Geometry: final body of the model. Coordinates: model frame, mm. A direction names the side the tool comes from. Give positions to 0.01 mm unless a question says otherwise; leave off trailing zeros. Loops run counter-clockwise (first coordinate to the right, second up) from the corner with the lowest first, then second, coordinate; pieces in that order, holes last. Notation, with made-up numbers: (68, 88.5) - (127, 88.5) arc R27 ccw to (127, 112.5) - close; hole circle Ø6 at (-32, 21.5). An arc over 180 degrees is marked (long way). Use one line per item in the form item = value.
Autodesk Inventor part; units mm, degrees
ref_plane "YZ Plane" through (0, 0, 0) normal (1, 0, 0) x (0, 1, 0)
ref_plane "XZ Plane" through (0, 0, 0) normal (0, 1, 0) x (-1, 0, 0)
ref_plane "XY Plane" through (0, 0, 0) normal (0, 0, 1) x (1, 0, 0)
sketch "Sketch1" plane through (0, 0, 0) normal (0, 0, 1) x (1, 0, 0)
  line L0 (0, 0) -> (0, 87.5)
  line L1 (0, 87.5) -> (43.6046, 111.967)
  line L2 (0, 0) -> (50, 0)
  line L3 (50, 0) -> (93.217, 25.1454)
  circle A0 centre (68.0717, 68.3624) radius 50 construction
  arc A1 (93.217, 25.1454) -> (43.6046, 111.967) centre (68.0717, 68.3624) ccw
  dimension "d0" = 87.5
  dimension "d1" = 50
  dimension "d2" = 50
  dimension "d3" = 50
  dimension "d4" = 100
extrude "Extrusion1" add sketch "Sketch1" along normal blind 50
sketch "Sketch2" plane through (0, 0, 50) normal (0, 0, 1) x (1, 0, 0)
  line L0 (0, 0) -> (50, 0)
  line L1 (50, 0) -> (93.217, 25.1454)
  arc A0 (93.217, 25.1454) -> (43.6046, 111.967) centre (68.0717, 68.3624) ccw
  line L2 (43.6046, 111.967) -> (0, 87.5)
  line L3 (0, 81.7667) -> (46.0513, 107.6066)
  arc A1 (90.7025, 29.4671) -> (46.0513, 107.6066) centre (68.0717, 68.3624) ccw
  line L4 (90.7025, 29.4671) -> (48.6512, 5)
  line L5 (48.6512, 5) -> (0, 5)
  line L6 (0, 87.5) -> (0, 0)
  line L7 (0, 5) -> (0, 81.7667)
  dimension "d7" = 5
extrude "Extrusion2" cut sketch "Sketch2" against normal blind 45 contours L6 L3 A1 L4 L5
sketch "Sketch3" plane through (0, 0, 0) normal (-1, 0, 0) x (0, 0, 1)
  line L0 (0, 87.5) -> (50, 87.5)
  line L1 (50, 113.3624) -> (50, 29.4671)
  line L2 (0, 87.5) -> (50, 87.5)
  line L3 (50, 87.5) -> (50, 72.5)
  line L4 (50, 72.5) -> (0, 72.5)
  line L5 (0, 72.5) -> (0, 87.5)
  point P0 (0, 0)
  point P1 (50, 107.6066)
  dimension "d10" = 15
extrude "Extrusion3" add sketch "Sketch3" against normal blind 5
sketch "Sketch4" plane through (0, 0, 0) normal (-1, 0, 0) x (0, 0, 1)
  line L0 (0, 87.5) -> (0, 111.967)
  line L1 (0, 87.5) -> (15, 87.5)
  line L2 (15, 87.5) -> (15, 32.5)
  line L3 (15, 32.5) -> (0, 32.5)
  line L4 (0, 32.5) -> (0, 87.5)
  line L5 (0, 0) -> (50, 0)
  dimension "d13" = 15
  dimension "d14" = 32.5
extrude "Extrusion4" add sketch "Sketch4" against normal blind 5
sketch "Sketch5" plane through (0, 0, 5) normal (0, 0, 1) x (1, 0, 0)
  circle A0 centre (25, 27.5) radius 5
  line L0 (0, 0) -> (50, 0)
  dimension "d17" = 10
  dimension "d18" = 27.5
  dimension "d19" = 25
extrude "Extrusion5" add sketch "Sketch5" along normal blind 90
sketch "Sketch6" plane through (0, 0, 5) normal (0, 0, 1) x (1, 0, 0)
  circle A0 centre (25, 27.5) radius 5
  circle A1 centre (25, 27.5) radius 20
  point P0 (0, 0)
  dimension "d22" = 40
extrude "Extrusion6" add sketch "Sketch6" along normal blind 10
sketch "Sketch7" plane through (0, 0, 5) normal (0, 0, 1) x (1, 0, 0)
  arc A0 (93.217, 25.1454) -> (43.6046, 111.967) centre (68.0717, 68.3624) ccw
  circle A1 centre (68.0717, 68.3624) radius 6.25
  circle A2 centre (68.0717, 68.3624) radius 21.25
  point P0 (0, 0)
  dimension "d25" = 12.5
  dimension "d28" = 15
extrude "Extrusion8" add sketch "Sketch7" along normal blind 10
sketch "Sketch8" plane through (68.0717, 68.3624, 5) normal (0, 0, 1) x (1, 0, 0)
  circle A0 centre (0, 0) radius 6.25
  circle A1 centre (0, 0) radius 6.25
  point P0 (-68.0717, -68.3624)
extrude "Extrusion9" cut sketch "Sketch8" against normal through all
sketch "Sketch9" plane through (0, 0, 0) normal (0, 0, -1) x (-1, 0, 0)
  circle A0 centre (-68.0717, 68.3624) radius 21.25
  circle A1 centre (-68.0717, 68.3624) radius 21.25
  point P0 (0, 0)
extrude "Extrusion10" add sketch "Sketch9" along normal blind 5
sketch "Sketch10" plane through (0, 0, 50) normal (0, 0, 1) x (1, 0, 0)
  arc A0 (93.217, 25.1454) -> (43.6046, 111.967) centre (68.0717, 68.3624) ccw
  circle A1 centre (68.0717, 68.3624) radius 50
  line L0 (18.0717, 68.3624) -> (18.0717, 97.6402)
  line L1 (0, 87.5) -> (43.6046, 111.967)
  line L2 (43.6046, 111.967) -> (18.0717, 97.6402)
  line L3 (68.0717, 18.3624) -> (81.5592, 18.3624)
  line L4 (50, 0) -> (93.217, 25.1454)
  line L5 (81.5592, 18.3624) -> (93.217, 25.1454)
  point P0 (0, 0)
extrude "Extrusion11" cut sketch "Sketch10" against normal blind 10
properties part number "BA005" material "ABS Plastic"
(1) Pin query (flat end, axial travel): P1, Ø1.5, axis at x = 88.5, y = 98, coming from the -Z side; P2, Ø8, axis at x = 57, z = 41, coming from the +Y side; P3, Ø3, axis at x = 74.5, z = 45, coming from the +Y side. Return the tip coordinate at first contact, or that it passes through.
Solution:
P1 = 0
P2 = 117.84
P3 = 18.36
(2) Pull-direction query (X, two-part tool) for faces 1 (the face through (111, 94, 20)), 2 (the face through (25.24, 95.93, 22.82)), 3 (the face through (0, 43, 14)); classes: released by +X, released by -X, zero draft, split by the parting line, or undercut.
Solution:
face_1 = split by the parting line
face_2 = undercut
face_3 = released by -X
(3) Cut plane C-C (y = 27.5). Return the cut outline in (x, z), plus the area to 3 significant figures.
Solution:
outline = (0, 0) - (96.89, 0) - (96.89, 40) - (87.32, 40) - (87.32, 5) - (45, 5) - (45, 15) - (30, 15) - (30, 95) - (20, 95) - (20, 15) - (5, 15) - (5, 5) - (0, 5) - close
area = 2,020 mm2
(4) Cut plane B-B (x = 55). Return the cut outline in (y, z), plus the area to 3 significant figures.
Solution:
outline = (2.91, 0) - (51.61, 0) - (51.61, -5) - (85.12, -5) - (85.12, 0) - (116.62, 0) - (116.62, 40) - (111.42, 40) - (111.42, 5) - (85.12, 5) - (85.12, 15) - (51.61, 15) - (51.61, 5) - (8.69, 5) - (8.69, 50) - (2.91, 50) - close
area = 1,510 mm2
(5) Cut plane A-A (z = 44). Return the cut outline in (x, y), plus the area to 3 significant figures.
Solution:
outline = (0, 0) - (50, 0) - (81.56, 18.36) - (71.62, 18.36) - (48.65, 5) - (0, 5) - close; (0, 72.5) - (5, 72.5) - (5, 84.57) - (18.07, 91.91) - (18.07, 97.64) - (0, 87.5) - close; circle Ø10 at (25, 27.5)
area = 640 mm2
(6) Access query for faces 4 (the face through (25, 5, 28)), 5 (the face through (77, 18.362, 45)), 6 (the face through (71.31, 12.4, 24.65)), 7 (the face through (47.803, 61.979, -2.465)), 8 (the face through (21, 30.5, 54.4)). Directions: +Z, -Z, +X, -X, +Y, -Y. A direction counts if a zero-diameter tool reaches every point of the face in a straight line with its end or side. Return the directions, or none.
Solution:
face_4 = +Z, -X
face_5 = +Z, +X, -X, +Y
face_6 = +Z, -Z, +X, -Y
face_7 = -Z
face_8 = +Z
(7) Cut plane D-D (z = 3). Return the cut outline in (x, y), plus the area to 3 significant figures.
Solution:
outline = (0, 0) - (50, 0) - (93.22, 25.15) arc R50 ccw to (43.6, 111.97) - (0, 87.5) - close; hole circle Ø12.5 at (68.07, 68.36)
area = 11,000 mm2
(8) Material intervals for L1, parallel to Y at x = 34, z = 14; L2, parallel to Y at x = 49, z = 9; L3, parallel to Y at x = 47, z = 48.5, sorted ascending. Write a range as from..to.
Solution:
L1 = 0..5, 9.64..45.36, 100.84..106.58
L2 = 0..5.2, 58.99..77.73, 109.12..114.58
L3 = 0..5
